```python
from build123d import *

# Parameters (mm, degrees)
BOSS_EXTRUDE1_DEPTH = 2.5
BOSS_EXTRUDE2_DEPTH = 12.5
SKETCH5_W           = 30.5
SKETCH5_H           = 6
BOSS_EXTRUDE3_DEPTH = 3.5
SKETCH6_W           = 6
SKETCH6_H           = 30.5
BOSS_EXTRUDE4_DEPTH = 3.5
CUT_EXTRUDE1_REACH  = 51.102
SKETCH3_R           = 2.75
CUT_EXTRUDE2_REACH  = 51.102
SKETCH4_R           = 2.75
FILLET1_R           = 8
CHAMFER1_SIZE       = 3


with BuildPart() as part:
    # Sketch1 → Boss-Extrude1 (new body)
    with BuildSketch(Plane.XY):
        Polygon((0, 0), (0, 35), (4, 35), (35, 4), (35, 0), align=None)
    extrude(amount=BOSS_EXTRUDE1_DEPTH)

    # Sketch2 → Boss-Extrude2 (add)
    with BuildSketch(Plane.XY.offset(2.5)):
        Polygon((35, 0), (35, 4), (4, 4), (4, 35), (0, 35), (0, 0), align=None)
    extrude(amount=BOSS_EXTRUDE2_DEPTH)

    # Sketch5 → Boss-Extrude3 (add)
    with BuildSketch(Plane.XZ):
        with Locations((19.75, 7.5)):
            Rectangle(SKETCH5_W, SKETCH5_H)
    extrude(amount=BOSS_EXTRUDE3_DEPTH)

    # Sketch6 → Boss-Extrude4 (add)
    with BuildSketch(Plane.ZY):
        with Locations((7.5, 19.75)):
            Rectangle(SKETCH6_W, SKETCH6_H)
    extrude(amount=BOSS_EXTRUDE4_DEPTH)

    # Sketch3 → Cut-Extrude1 (cut, up to next)
    with BuildSketch(Plane(origin=(4, 0, 0), x_dir=(0, 0, -1), z_dir=(1, 0, 0)), mode=Mode.PRIVATE) as cut_extrude1_sk1:
        with Locations((-7.5, 23.5)):
            Circle(SKETCH3_R)
    cut_extrude1_tool1 = extrude(cut_extrude1_sk1.sketch, amount=-CUT_EXTRUDE1_REACH, mode=Mode.PRIVATE) & part.part
    add(cut_extrude1_tool1.solids().sort_by_distance((4, 23.5, 7.5))[0], mode=Mode.SUBTRACT)

    # Sketch4 → Cut-Extrude2 (cut, up to next)
    with BuildSketch(Plane(origin=(0, 4, 0), x_dir=(1, 0, 0), z_dir=(0, 1, 0)), mode=Mode.PRIVATE) as cut_extrude2_sk1:
        with Locations(Location((23.5, -7.5, 0), (0, 0, 270))):
            Circle(SKETCH4_R)
    cut_extrude2_tool1 = extrude(cut_extrude2_sk1.sketch, amount=-CUT_EXTRUDE2_REACH, mode=Mode.PRIVATE) & part.part
    add(cut_extrude2_tool1.solids().sort_by_distance((23.5, 4, 7.5))[0], mode=Mode.SUBTRACT)

    # Fillet1
    fillet1_edges = [part.edges().sort_by_distance(p)[0] for p in [
        (4, 4, 8.75),
    ]]
    fillet(fillet1_edges, radius=FILLET1_R)

    # Chamfer1
    chamfer1_edges = [part.edges().sort_by_distance(p)[0] for p in [
        (0, 0, 7.5),
    ]]
    chamfer(chamfer1_edges, length=CHAMFER1_SIZE)


solid = part.part
```
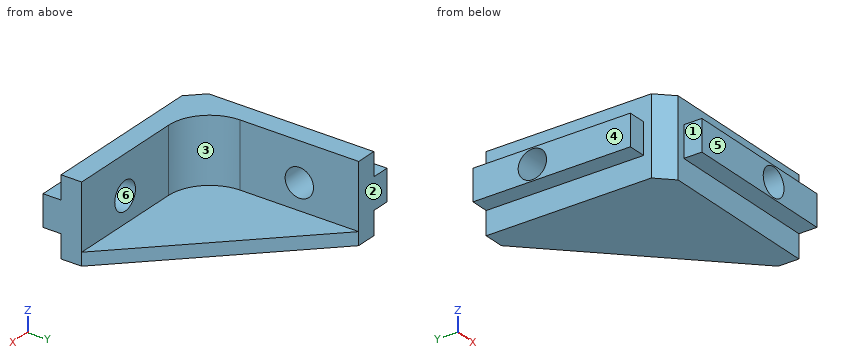
Geometry check sheet. Reference: the model listing, model coordinates, mm. Face numbers are marked on the shaded views. A direction names the side the tool comes from. Coordinates: 2 decimals unless noted, no trailing zeros. Loops run counter-clockwise (first coordinate to the right, second up) from the corner with the lowest first, then second, coordinate; pieces in that order, holes last.
Item 1: Sectioned sample at A-A, the plane y = 23.5. Record the boundary of the cut face in (x, z), then the cut area to 3 significant figures.
Item 2: Access from +Z, -Z, +X, -X, +Y, -Y to the whole of each face (thin tool, end or side, straight path). Record for the marked faces 1, 2 and 3.
Item 3: Thickness scan on line 1 (Y direction, x = -0.25, z = 7.5); line 2 (Y direction, x = 22, z = 10.25). Record the ranges inside material, lowest first.
Item 4: Sectioned sample at D-D, the plane y = 16. Record the boundary of the cut face in (x, z), then the cut area to 4 significant figures.
Item 5: Go/stop test with flat-tipped pins: pin 1 Ø3 at (x, y) = (25.5, -2) entering from -Z; pin 2 Ø1 at (x, y) = (1.5, 23) entering from -Z; pin 3 Ø4.5 at (x, z) = (23.5, 7.5) entering from -Y; pin 4 Ø1 at (x, z) = (-1.5, 7) entering from -Y. Record where each tip stops, or that it passes through.
Item 6: Release check for a two-part mould opening along X. For the marked faces 4, 5 and 6 record: released by +X, released by -X, zero draft, split by the parting line, or undercut.
Item 7: Sectioned sample at C-C, the plane z = 7.5. Record the boundary of the cut face in (x, y).
Check result:
1. outline: (-3.5, 4.5) - (0, 4.5) - (0, 0) - (15.5, 0) - (15.5, 2.5) - (4, 2.5) - (4, 4.75) - (-3.5, 4.75) - close; (-3.5, 10.25) - (4, 10.25) - (4, 15) - (0, 15) - (0, 10.5) - (-3.5, 10.5) - close
1. area: 68.5 mm2
2. face 1: +Z, -Z, -X, -Y
2. face 2: +Z, -Z, +X, -X, +Y
2. face 3: +Z, +X, +Y
3. line 1: y = 4.5 to 20.75, 26.25 to 35
3. line 2: y = -3.5 to 4
4. outline: (-3.5, 4.5) - (0, 4.5) - (0, 0) - (23, 0) - (23, 2.5) - (4, 2.5) - (4, 15) - (0, 15) - (0, 10.5) - (-3.5, 10.5) - close
4. area: 128.5 mm2
5. pin 1: stops at z = 4.5
5. pin 2: stops at z = 0
5. pin 3: passes through
5. pin 4: stops at y = 4.5
6. face 4: released by -X
6. face 5: zero draft
6. face 6: undercut
7. outline: (-3.5, 4.5) - (0, 4.5) - (0, 3) - (3, 0) - (4.5, 0) - (4.5, -3.5) - (20.75, -3.5) - (20.75, 4) - (12, 4) arc R8 cw to (4, 12) - (4, 20.75) - (-3.5, 20.75) - close; (-3.5, 26.25) - (4, 26.25) - (4, 35) - (-3.5, 35) - close; (26.25, -3.5) - (35, -3.5) - (35, 4) - (26.25, 4) - close
